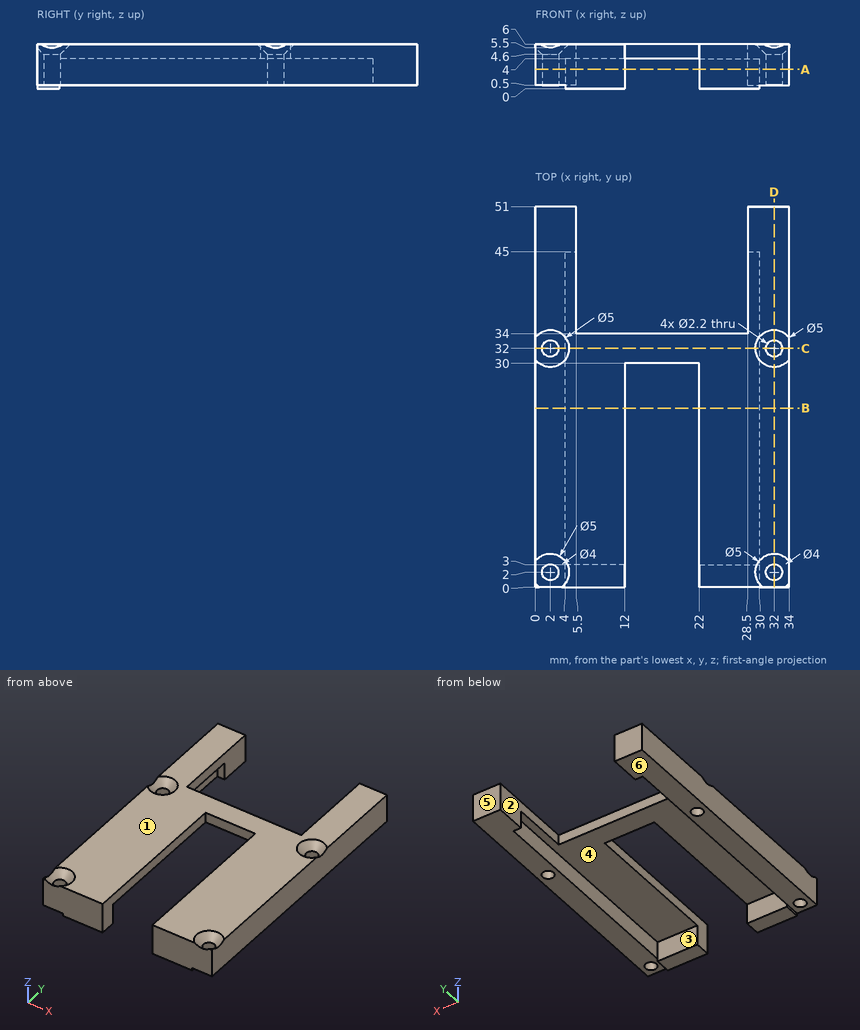
The figure shows three views and two pictorial views of one solid part (mm, origin at its lowest corner). Answer the questions. A direction names the side the tool comes from. Coordinates: 2 decimals unless noted, no trailing zeros. Write each loop counter-clockwise with the first axis right and the second up, starting at its lowest first coordinate (ties: lowest second). Pieces come first, ordered by that corner, then holes. Notation, with made-up numbers: (81, 88.5) -> (90, 88.5) arc R24 cw to (90, 112.5) -> close; hole circle Ø1 at (-2.5, 16). An arc over 180 degrees is marked (long way). Return JSON: item names as keys, results as strings.
(1) The part is cut by section B-B on y = 24. Give the vertices of the cut face in (x, z).
Answers below:
{"outline": "(0, 0.5) -> (4, 0.5) -> (4, 4) -> (12, 4) -> (12, 6) -> (0, 6) -> close; (22, 4) -> (30, 4) -> (30, 0.5) -> (34, 0.5) -> (34, 6) -> (22, 6) -> close"}
(2) The part is cut by section A-A on z = 2.6. Give the vertices of the cut face in (x, y), then the cut area to 3 significant figures.
Answers below:
{"outline": "(0, 0) -> (12, 0) -> (12, 3) -> (4, 3) -> (4, 45) -> (5.5, 45) -> (5.5, 51) -> (0, 51) -> close; (22, 0) -> (34, 0) -> (34, 51) -> (28.5, 51) -> (28.5, 45) -> (30, 45) -> (30, 3) -> (22, 3) -> close; hole circle Ø2.2 at (2, 2); hole circle Ø2.2 at (2, 32); hole circle Ø2.2 at (32, 2); hole circle Ø2.2 at (32, 32)", "area": "459 mm^2"}
(3) For a pull along Y with two mould halves and no side action, classify the marked faces 4, 5 and 6 as pulls with the +Y half, pulls with the -Y half, needs draft (parallel to the pull), parting line crosses it, or undercut.
Answers below:
{"face 4": "undercut", "face 5": "pulls with the +Y half", "face 6": "needs draft"}
(4) The part is cut by section D-D on x = 32. Give the vertices of the cut face in (y, z).
Answers below:
{"outline": "(0, 0.5) -> (0.9, 0.5) -> (0.9, 4.6) -> (0, 5.5) -> close; (3.1, 0.5) -> (30.9, 0.5) -> (30.9, 4.6) -> (29.5, 6) -> (4.5, 6) -> (3.1, 4.6) -> close; (33.1, 0.5) -> (51, 0.5) -> (51, 6) -> (34.5, 6) -> (33.1, 4.6) -> close"}
(5) Each of these flat-tipped pins is pushed along its axis until it touches: P1, Ø3, axis at x = 26.5, y = 14, coming from the -Z side; P2, Ø4, axis at x = 30.5, y = 20.5, coming from the -Z side; P3, Ø1.3, axis at x = 2, y = 2, coming from the -Z side; P4, Ø3.5, axis at x = 32, y = 2, coming from the +Z side. Where does it stop, or does it pass through?
Answers below:
{"P1": "z = 4", "P2": "z = 0.5", "P3": "through", "P4": "z = 5.25"}
(6) The part is cut by section C-C on y = 32. Give the vertices of the cut face in (x, z).
Answers below:
{"outline": "(0, 0.5) -> (0.9, 0.5) -> (0.9, 4.6) -> (0, 5.5) -> close; (3.1, 0.5) -> (4, 0.5) -> (4, 4) -> (30, 4) -> (30, 0.5) -> (30.9, 0.5) -> (30.9, 4.6) -> (29.5, 6) -> (4.5, 6) -> (3.1, 4.6) -> close; (33.1, 0.5) -> (34, 0.5) -> (34, 5.5) -> (33.1, 4.6) -> close"}
(7) Consider line 1 along Y through (x, z) = (2, 1.55); line 2 along X through (y, z) = (32, 2.2); line 3 along Y through (x, z) = (2.5, 3.1). Determine where each line is inside the solid, lowest interval first. Write a range as from..to.
Answers below:
{"line 1": "0..0.9, 3.1..30.9, 33.1..51", "line 2": "0..0.9, 3.1..4, 30..30.9, 33.1..34", "line 3": "0..1.02, 2.98..31.02, 32.98..51"}
(8) Which of the six approach directions +Z, -Z, +X, -X, +Y, -Y give full straight-line access (tool end or side, diameter ignored) to the marked faces 1, 2 and 3?
Answers below:
{"face 1": "+Z, +X, -X, +Y, -Y", "face 2": "+Z, -Z, +Y", "face 3": "-Z"}
